Autodesk Inventor part; units mm, degrees
ref_plane "YZ Plane" through (0, 0, 0) normal (1, 0, 0) x (0, 1, 0)
ref_plane "XZ Plane" through (0, 0, 0) normal (0, 1, 0) x (-1, 0, 0)
ref_plane "XY Plane" through (0, 0, 0) normal (0, 0, 1) x (1, 0, 0)
sketch "Sketch1" plane through (0, 0, 0) normal (0, 0, 1) x (1, 0, 0)
  line L0 (160.3375, -152.4) -> (-160.3375, -152.4)
  line L1 (-160.3375, -152.4) -> (-160.3375, 0)
  line L2 (-160.3375, 0) -> (160.3375, 0)
  line L3 (160.3375, 0) -> (160.3375, -152.4)
  line L4 (0, 223.4715) -> (0, -292.8328)
  line L5 (-302.26, 0) -> (302.26, 0)
  line L6 (215.9, -219.075) -> (-215.9, -219.075)
  line L7 (-215.9, -219.075) -> (-215.9, -152.4)
  line L8 (-215.9, -152.4) -> (215.9, -152.4)
  line L9 (215.9, -152.4) -> (215.9, -219.075)
  line L10 (215.9, -219.075) -> (-215.9, -152.4) construction
  line L11 (-215.9, -219.075) -> (215.9, -152.4) construction
  line L12 (0, 0) -> (0, 149.7138) construction
  line L13 (-143.6687, -198.12) -> (-186.5312, -198.12) construction
  line L14 (76.2, -105.41) -> (-76.2, -105.41) construction
  line L15 (-76.2, -105.41) -> (-76.2, -123.19) construction
  line L16 (-76.2, -123.19) -> (76.2, -123.19) construction
  line L17 (76.2, -123.19) -> (76.2, -105.41) construction
  line L18 (76.2, -105.41) -> (-76.2, -123.19) construction
  line L19 (-76.2, -105.41) -> (76.2, -123.19) construction
  point P0 (0, -185.7375)
  point P1 (-165.1, -198.12)
  point P2 (0, -114.3)
  point P3 (114.3, -114.3)
  point P4 (-114.3, -114.3)
  point P5 (0, -114.3)
  point P6 (-146.05, -114.3)
  point P7 (146.05, -114.3)
  point P8 (0, -114.3)
  point P9 (0, -114.3)
  dimension "d0" = 320.675
  dimension "d2" = 66.675
  dimension "d3" = 431.8
  dimension "d5" = 152.4
  dimension "d6" = 0
  dimension "d7" = 0
  dimension "d10" = 42.8625
  dimension "d11" = 165.1
  dimension "d12" = 29.3687
  dimension "d24" = 17.78
  dimension "d25" = 152.4
  dimension "d26" = 114.3
  dimension "d27" = 114.3
  dimension "d28" = 114.3
  dimension "d50" = 198.12
  dimension "d55" = 31.75
  dimension "d56" = 31.75
extrude "Extrusion1" add sketch "Sketch1" along normal blind 9.144
hole "Hole1-Regulator Brkt Mtg" at (-186.5312, -198.12, 0) at (-143.6687, -198.12, 0) direction (0, 0, 1) diameter 4.1402 end through all
pattern_linear "Rectangular Pattern1" count 5 spacing 82.55 along (1, 0, 0) of "Hole1-Regulator Brkt Mtg"
sketch "Sketch2" plane through (0, 0, 9.144) normal (0, 0, 1) x (1, 0, 0)
  circle A0 centre (186.5313, -198.12) radius 2.0701
  line L0 (215.9, -219.075) -> (215.9, -152.4)
  point P0 (0, 0)
  dimension "d23" = 29.3687
hole "Hole2-Manifold Mtg" at (-114.3, -114.3, 0) at (-76.2, -123.19, 0) at (76.2, -105.41, 0) at (114.3, -114.3, 0) at (0, -114.3, 0) at (-146.05, -114.3, 0) at (146.05, -114.3, 0) direction (0, 0, 1) diameter 3.2512 end through all
sketch "Sketch3" plane through (0, 0, 0) normal (0, 0, 1) x (1, 0, 0)
  line L0 (-101.6, -15.24) -> (101.6, -15.24) construction
  line L1 (-203.2, -167.64) -> (203.2, -167.64) construction
  line L2 (0, 0) -> (0, 149.7138) construction
  line L3 (0, 223.4715) -> (0, -292.8328) construction
  line L4 (-287.02, 0) -> (299.72, 0) construction
  point P0 (0, -15.24)
  point P1 (0, -167.64)
  dimension "d36" = 101.6
  dimension "d37" = 101.6
  dimension "d38" = 15.24
  dimension "d39" = 203.2
  dimension "d40" = 406.4
  dimension "d41" = 152.4
  dimension "d54" = 152.4
hole "Hole3-Mount to Base plate" at (-101.6, -15.24, 0) at (101.6, -15.24, 0) at (203.2, -167.64, 0) at (-203.2, -167.64, 0) at (0, -15.24, 0) at (0, -167.64, 0) direction (0, 0, 1) diameter 7.493 end through all
fillet "Fillet1" radius 6.35 8 edges at (-215.9, -219.075, 4.572) (215.9, -219.075, 4.572) (160.3375, 0, 4.572) (160.3375, -152.4, 4.572) (215.9, -152.4, 4.572) (-215.9, -152.4, 4.572) (-160.3375, -152.4, 4.572) (-160.3375, 0, 4.572)
pattern_linear "Rectangular Pattern2" count 3 spacing 38.1 along (0, 1, 0) of "Hole2-Manifold Mtg"
sketch "Sketch4" plane through (0, 0, 0) normal (0, 0, 1) x (1, 0, 0)
  circle A0 centre (-143.6687, -198.12) radius 2.0701
  circle A1 centre (-103.9812, -198.12) radius 2.0701
  circle A2 centre (-143.6687, -198.12) radius 2.0701 construction
  circle A3 centre (-103.9812, -198.12) radius 2.0701 construction
  line L0 (-143.6687, -198.12) -> (-103.9812, -198.12) construction
  line L1 (-123.8599, -207.645) -> (-123.825, -198.12) construction
  line L2 (0, 43.815) -> (0, -262.89)
  point P0 (0, 0)
  point P1 (-123.8599, -55.245)
  point P2 (-123.8599, -17.145)
  dimension "d57" = 152.4
  dimension "d58" = 38.1
  dimension "d66" = 9.525
  dimension "d67" = 123.8599
hole "Hole4-trough mounting" at (-123.8599, -17.145, 0) at (-123.8599, -55.245, 0) at (-123.8599, -207.645, 0) direction (0, 0, 1) diameter 3.2512 end through all
mirror "Mirror1" about plane through (0, 0, 0) normal (1, 0, 0) of "Hole4-trough mounting"
pattern_linear "Rectangular Pattern3" count 2 spacing 123.8504 along (1, 0, 0) of "Hole4-trough mounting"
properties part number "J005209"
The listing builds one solid part. Answer for the finished solid, in the listing's coordinates (mm). A direction names the side the tool comes from. Round coordinates to 2 decimals unless told otherwise and drop trailing zeros. Return JSON: item names as keys, results as strings. Group by question number.
1. The part is cut by section A-A on z = 3.5. State how many separate pieces and enclosed holes the cut face has, then the cut area to 3 significant figures.
2. The mould has two halves that part along Y. Classify faces 4 (the flat face through (215.9, -185, 5)), 5 (the flat face through (-188, -152.4, 5)), 6 (the cylindrical face through (-1.13, -164.07, 4.64)): pulls with the +Y half, pulls with the -Y half, needs draft (parallel to the pull), parting line crosses it, or undercut.
3. Consider probe 1 along X at (y, z) = (-76.2, 3.5); probe 2 along Y at (x, z) = (114.3, 5.5) (3 decimals); probe 3 along X at (y, z) = (-167.64, 4.75). Determine where each line is inside the solid, lowest interval first.
4. This flat-tipped pin is pushed along its axis until it touches: P1, Ø3, axis at y = -75, z = 2.5, coming from the -X side. Where does it stop, or does it pass through?
5. Which of the six approach directions +Z, -Z, +X, -X, +Y, -Y give full straight-line access (tool end or side, diameter ignored) to faces 1 (the flat face through (-160.338, -77, 5)), 2 (the flat face through (188, -152.4, 5)), 3 (the flat face through (-2, 0, 5))?
Resolved:
{
 "1": {"separate pieces": "1", "enclosed holes": "45", "area": "77,000 mm²"},
 "2": {"face 4": "needs draft", "face 5": "pulls with the +Y half", "face 6": "undercut"},
 "3": {"probe 1": "x = -160.34 to -147.68, -144.42 to -115.93, -112.67 to -1.63, 1.63 to 112.67, 115.93 to 144.42, 147.68 to 160.34", "probe 2": "y = -219.075 to -115.926, -112.674 to -77.826, -74.574 to -39.726, -36.474 to 0", "probe 3": "x = -215.9 to -206.95, -199.45 to -3.75, 3.75 to 199.45, 206.95 to 215.9"},
 "4": {"P1": "stops at x = -160.34"},
 "5": {"face 1": "+Z, -Z, -X, +Y", "face 2": "+Z, -Z, +X, +Y", "face 3": "+Z, -Z, +X, -X, +Y"}
}
